Can you work these out from the model? Positions are in its coordinate system, mm. Give positions to 0.01 mm unless a question says otherwise; leave off trailing zeros. Order: outer loops, then holes, each group sorted by start corner. A loop starts at its lowest first (then second) coordinate and runs counter-clockwise, first axis right, second up. Notation, with made-up numbers: (86, -28.75) - (133, -28.75) arc R24 ccw to (133, -11.75) - close; hole circle Ø3 at (37, -15). An arc over 180 degrees is marked (long way). Answer as CSV lines item,"result".
```python
from build123d import *

# Parameters (mm, degrees)
BOSS_EXTRUDE1_DEPTH = 2.286
SKETCH3_R           = 2.4638
CUT_EXTRUDE2_DEPTH  = 126.744366856


with BuildPart() as part:
    # Sketch1 → Boss-Extrude1 (new body)
    with BuildSketch(Plane(origin=(0, 0, 0), x_dir=(1, 0, 0), z_dir=(0, 1, 0))):
        Polygon((25.4, 38.1), (38.1, 25.4), (88.9, 25.4), (88.9, 0), (0, 0), (0, 88.9), (25.4, 88.9), align=None)
    boss_extrude1 = extrude(amount=BOSS_EXTRUDE1_DEPTH)

    # Mirror1: Boss-Extrude1 across plane
    add(boss_extrude1.mirror(Plane.ZY.offset(-12.7)))

    # Sketch3 → Cut-Extrude2 (cut, through all)
    with BuildSketch(Plane(origin=(0, 2.286, 0), x_dir=(1, 0, 0), z_dir=(0, 1, 0))):
        with Locations(Location((76.2, 12.7, 0), (0, 0, 270))):
            Circle(SKETCH3_R)
        with Locations(Location((12.7, 12.7, 0), (0, 0, 270))):
            Circle(SKETCH3_R)
        with Locations(Location((12.7, 76.2, 0), (0, 0, 270))):
            Circle(SKETCH3_R)
        with Locations(Location((12.7, 38.1, 0), (0, 0, 270))):
            Circle(SKETCH3_R)
        with Locations(Location((38.1, 12.7, 0), (0, 0, 270))):
            Circle(SKETCH3_R)
    cut_extrude2 = extrude(amount=-CUT_EXTRUDE2_DEPTH, mode=Mode.SUBTRACT)

    # Mirror2: Cut-Extrude2 across plane
    add(cut_extrude2.mirror(Plane.ZY.offset(-12.7)), mode=Mode.SUBTRACT)


solid = part.part
```
1) I want a section at C-C on x = 12.7. Write out the boundary of the cut face in (y, z).
Answer block:
outline,"(0, -88.9) - (2.29, -88.9) - (2.29, -78.66) - (0, -78.66) - close; (0, -73.74) - (2.29, -73.74) - (2.29, -40.56) - (0, -40.56) - close; (0, -35.64) - (2.29, -35.64) - (2.29, -15.16) - (0, -15.16) - close; (0, -10.24) - (2.29, -10.24) - (2.29, 0) - (0, 0) - close"
2) I want a section at D-D on z = -12.7. Write out the boundary of the cut face in (x, y).
Answer block:
outline,"(-63.5, 0) - (-53.26, 0) - (-53.26, 2.29) - (-63.5, 2.29) - close; (-48.34, 0) - (-15.16, 0) - (-15.16, 2.29) - (-48.34, 2.29) - close; (-10.24, 0) - (10.24, 0) - (10.24, 2.29) - (-10.24, 2.29) - close; (15.16, 0) - (35.64, 0) - (35.64, 2.29) - (15.16, 2.29) - close; (40.56, 0) - (73.74, 0) - (73.74, 2.29) - (40.56, 2.29) - close; (78.66, 0) - (88.9, 0) - (88.9, 2.29) - (78.66, 2.29) - close"
3) I'm going to push flat-ended pins straight in: P1, Ø3, axis at x = -12.7, z = -12.7, coming from the +Y side; P2, Ø1.1, axis at y = 1, z = -66.5, coming from the +X side; P3, Ø0.7, axis at x = 65, y = 0.5, coming from the -Z side; P4, Ø1.1, axis at y = 1.5, z = -76, coming from the -X side. Where does each tip first touch, or does it pass through?
Answer block:
P1,"through"
P2,"x = 25.4"
P3,"z = -25.4"
P4,"x = 0"
4) If we mould it in two halves opening along X, with no side actions, what happens to faces 1 (the cylindrical face through (11.201, 1.159, -40.055)), 2 (the flat face through (31.7, 1.1, -31.8)), 3 (the flat face through (12, 2.286, -25))? For each: +X half, -X half, draft (parallel to the pull), parting line (faces both ways), or undercut.
Answer block:
face 1,"undercut"
face 2,"+X half"
face 3,"draft"
5) I need wall thicknesses on line 1 along X through (y, z) = (1.1, -12.7); line 2 along X through (y, z) = (1.7, -10.5); line 3 along Z through (x, y) = (-50.8, 0.6). Which ranges of each line are inside material? Lowest first, please. Write a range as [from, to].
Answer block:
line 1,"[-63.5, -53.26], [-48.34, -15.16], [-10.24, 10.24], [15.16, 35.64], [40.56, 73.74], [78.66, 88.9]"
line 2,"[-63.5, -51.91], [-49.69, -13.81], [-11.59, 11.59], [13.81, 36.99], [39.21, 75.09], [77.31, 88.9]"
line 3,"[-25.4, -15.16], [-10.24, 0]"
6) I want a section at A-A on x = -50.8. Write out the boundary of the cut face in (y, z).
Answer block:
outline,"(0, -25.4) - (2.29, -25.4) - (2.29, -15.16) - (0, -15.16) - close; (0, -10.24) - (2.29, -10.24) - (2.29, 0) - (0, 0) - close"
7) I want a section at B-B on z = -76.2. Write out the boundary of the cut face in (x, y), plus the area to 3 significant figures.
Answer block:
outline,"(0, 0) - (10.24, 0) - (10.24, 2.29) - (0, 2.29) - close; (15.16, 0) - (25.4, 0) - (25.4, 2.29) - (15.16, 2.29) - close"
area,"46.8 mm2"
